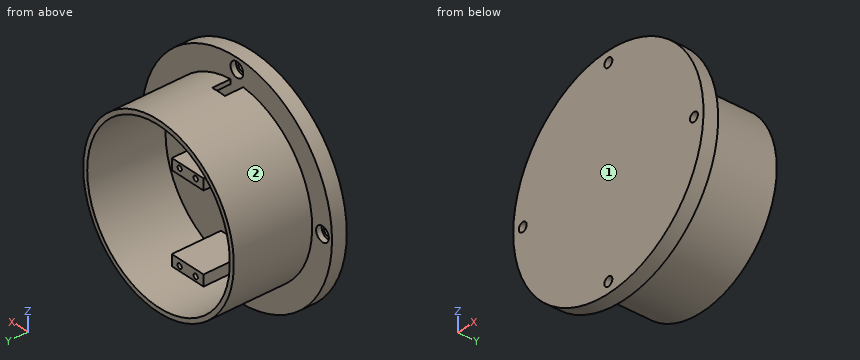
Autodesk Inventor part; units mm, degrees
ref_plane "YZ Plane" through (0, 0, 0) normal (1, 0, 0) x (0, 1, 0)
ref_plane "XZ Plane" through (0, 0, 0) normal (0, 1, 0) x (-1, 0, 0)
ref_plane "XY Plane" through (0, 0, 0) normal (0, 0, 1) x (1, 0, 0)
sketch "Sketch1" plane through (0, 0, 0) normal (0, 1, 0) x (-1, 0, 0)
  circle A0 centre (0, 0) radius 60
  dimension "d0" = 120
extrude "Extrusion1" add sketch "Sketch1" along normal blind 8
sketch "Sketch2" plane through (0, 8, 0) normal (0, 1, 0) x (1, 0, 0)
  circle A0 centre (-54, 0) radius 4
  circle A1 centre (-54, 0) radius 2.5
  circle A2 centre (0, -54) radius 4
  circle A3 centre (0, -54) radius 2.5
  circle A4 centre (54, 0) radius 4
  circle A5 centre (54, 0) radius 2.5
  circle A6 centre (0, 54) radius 4
  circle A7 centre (0, 54) radius 2.5
  point P0 (0, 0)
  dimension "d3" = 8
  dimension "d4" = 5
  dimension "d5" = 8
  dimension "d6" = 5
  dimension "d7" = 8
  dimension "d8" = 5
  dimension "d9" = 8
  dimension "d10" = 5
extrude "Extrusion2" cut sketch "Sketch2" against normal blind 8 contours A1 | A3 | A5 | A7
sketch "Sketch3" plane through (0, 8, 0) normal (0, 1, 0) x (1, 0, 0)
  circle A0 centre (-54, 0) radius 2.5
  circle A1 centre (-54, 0) radius 4
  circle A2 centre (-54, 0) radius 2.5
  circle A3 centre (0, 54) radius 2.5
  circle A4 centre (0, 54) radius 4
  circle A5 centre (0, 54) radius 2.5
  circle A6 centre (54, 0) radius 2.5
  circle A7 centre (54, 0) radius 4
  circle A8 centre (54, 0) radius 2.5
  circle A9 centre (0, -54) radius 4
  circle A10 centre (0, -54) radius 2.5
  point P0 (0, 0)
  dimension "d13" = 8
  dimension "d14" = 8
  dimension "d15" = 5
  dimension "d16" = 8
  dimension "d17" = 5
  dimension "d18" = 8
extrude "Extrusion3" cut sketch "Sketch3" against normal blind 3
sketch "Sketch4" plane through (0, 8, 0) normal (0, 1, 0) x (1, 0, 0)
  circle A0 centre (0, 0) radius 47.5
  circle A1 centre (0, 0) radius 45
  line L0 (0, 0) -> (-10, 0)
  line L1 (-10, 0) -> (-10, -9)
  line L2 (-10, -9) -> (0, -9)
  line L3 (0, -9) -> (0, 0)
  line L4 (0, -9) -> (10, -9)
  line L5 (10, -9) -> (10, 0)
  line L6 (10, 0) -> (0, 0)
  line L7 (0, 0) -> (0, -9)
  line L8 (-10, -9) -> (10, -9)
  line L9 (10, -9) -> (10, -16)
  line L10 (10, -16) -> (-10, -16)
  line L11 (-10, -16) -> (-10, -9)
  dimension "d21" = 95
  dimension "d22" = 90
  dimension "d23" = 10
  dimension "d24" = 9
  dimension "d25" = 10
  dimension "d26" = 7
extrude "Extrusion4" add sketch "Sketch4" along normal blind 10 contours A0
sketch "Sketch5" plane through (0, 8, 0) normal (0, 1, 0) x (1, 0, 0)
  line L0 (0, 0) -> (-10, 0)
  line L1 (-10, 0) -> (-10, -9)
  line L2 (-10, -9) -> (0, -9)
  line L3 (0, -9) -> (0, 0)
  line L4 (-10, -9) -> (10, -9)
  line L5 (10, -9) -> (10, -16)
  line L6 (10, -16) -> (-10, -16)
  line L7 (-10, -16) -> (-10, -9)
  line L8 (-10, -9) -> (10, -9)
  line L9 (10, -9) -> (10, 31)
  line L10 (10, 31) -> (-10, 31)
  line L11 (-10, 31) -> (-10, -9)
  line L12 (-10, 31) -> (-2, 31)
  line L13 (-2, 31) -> (-2, 38.36)
  line L14 (-2, 38.36) -> (-10, 38.36)
  line L15 (-10, 38.36) -> (-10, 31)
  line L16 (-10, 31) -> (10, 31)
  line L17 (10, 31) -> (10, 39)
  line L18 (10, 39) -> (-10, 39)
  line L19 (-10, 39) -> (-10, 31)
  line L20 (-10, -9) -> (10, -9)
  line L21 (10, -9) -> (10, -17)
  line L22 (10, -17) -> (-10, -17)
  line L23 (-10, -17) -> (-10, -9)
  dimension "d29" = 10
  dimension "d30" = 9
  dimension "d31" = 20
  dimension "d32" = 7
  dimension "d33" = 40
  dimension "d34" = 8
  dimension "d35" = 8
  dimension "d36" = 8
extrude "Extrusion5" add sketch "Sketch5" along normal blind 28 contours L4 L5 L6 L7 L2 | L15 L14 L13 L10 | L6 L21 L22 L23 | L13 L14 L19 L18 L17 L10
sketch "Sketch6" plane through (0, 36, 0) normal (0, 1, 0) x (1, 0, 0)
  line L0 (10, -17) -> (-10, -17)
  line L1 (-10, -9) -> (10, -9)
  line L2 (0, -17) -> (-4, -17)
  line L3 (-4, -17) -> (-4, -9)
  line L4 (-4, -9) -> (0, -9)
  line L5 (0, -9) -> (0, -17)
  line L6 (0, -17) -> (4, -17)
  line L7 (4, -17) -> (4, -9)
  line L8 (4, -9) -> (0, -9)
  line L9 (0, -9) -> (0, -17)
  point P0 (0, 0)
  dimension "d39" = 4
  dimension "d40" = 4
extrude "Extrusion6" cut sketch "Sketch6" against normal blind 28
sketch "Sketch7" plane through (0, 36, 0) normal (0, 1, 0) x (1, 0, 0)
  line L0 (-10, -17) -> (-4, -17)
  line L1 (4, -9) -> (10, -9)
  line L2 (-4, -17) -> (4, -17)
  line L3 (4, -17) -> (4, -9)
  line L4 (4, -9) -> (-4, -9)
  line L5 (-4, -9) -> (-4, -17)
  point P0 (0, 0)
extrude "Extrusion7" add sketch "Sketch7" against normal blind 22
sketch "Sketch8" plane through (0, 36, 0) normal (0, 1, 0) x (1, 0, 0)
  line L0 (-4, -17) -> (-10, -17)
  line L1 (10, -17) -> (10, -9)
  line L2 (-10, -17) -> (10, -17)
  line L3 (10, -17) -> (10, -15)
  line L4 (10, -15) -> (-10, -15)
  line L5 (-10, -15) -> (-10, -17)
  line L6 (-4, -9) -> (4, -9)
  line L7 (0, -9) -> (-5, -9)
  line L8 (-5, -9) -> (-5, -17)
  line L9 (-5, -17) -> (0, -17)
  line L10 (0, -17) -> (0, -9)
  line L11 (-10, -17) -> (10, -17)
  line L12 (0, -9) -> (5, -9)
  line L13 (5, -9) -> (5, -17)
  line L14 (5, -17) -> (0, -17)
  line L15 (0, -17) -> (0, -9)
  circle A0 centre (-5, -15) radius 2
  circle A1 centre (5, -15) radius 2
  line L16 (-10, 31) -> (-10, 39)
  line L17 (10, 39) -> (10, 31)
  line L18 (-10, 39) -> (10, 39)
  line L19 (10, 39) -> (10, 37)
  line L20 (10, 37) -> (-10, 37)
  line L21 (-10, 37) -> (-10, 39)
  line L22 (10, 31) -> (-10, 31)
  line L23 (-10, 39) -> (10, 39)
  line L24 (0, 31) -> (-5, 31)
  line L25 (-5, 31) -> (-5, 39)
  line L26 (-5, 39) -> (0, 39)
  line L27 (0, 39) -> (0, 31)
  line L28 (0, 31) -> (5, 31)
  line L29 (5, 31) -> (5, 39)
  line L30 (5, 39) -> (0, 39)
  line L31 (0, 39) -> (0, 31)
  circle A2 centre (-5, 37) radius 2
  circle A3 centre (5, 37) radius 2
  point P0 (0, 0)
  dimension "d45" = 2
  dimension "d46" = 5
  dimension "d47" = 5
  dimension "d48" = 4
  dimension "d49" = 4
  dimension "d50" = 2
  dimension "d51" = 4
  dimension "d52" = 4
extrude "Extrusion8" cut sketch "Sketch8" against normal blind 10 contours A0 L4 L8 | L8 L4 A0 | L8 A0 L4 | L4 A0 L8 | A1 L4 L13 | L13 L4 A1 | L13 A1 L4 | L4 A1 L13 | A2 L25 L20 | L20 L25 A2 | L25 L20 A2 | A2 L20 L25 | A3 L20 L29 | L29 L20 A3 | A3 L29 L20 | A3 L20 L29
sketch "Sketch9" plane through (0, 36, 0) normal (0, 1, 0) x (1, 0, 0)
  line L0 (-10, -17) -> (-5, -17)
  line L1 (10, -9) -> (-10, -9)
  line L2 (-10, -17) -> (10, -17)
  line L3 (10, -17) -> (10, -9)
  line L4 (10, -9) -> (-10, -9)
  line L5 (-10, -9) -> (-10, -17)
  line L6 (10, 31) -> (10, 39)
  line L7 (-10, 31) -> (10, 31)
  line L8 (10, 31) -> (10, 39)
  line L9 (10, 39) -> (-10, 39)
  line L10 (-10, 39) -> (-10, 31)
  point P0 (0, 0)
extrude "Extrusion9" cut sketch "Sketch9" against normal blind 28
sketch "Sketch10" plane through (0, 8, 0) normal (0, 1, 0) x (1, 0, 0)
  line L0 (0, 0) -> (-10, 0)
  line L1 (-10, 0) -> (-10, 36.5)
  line L2 (-10, 36.5) -> (0, 36.5)
  line L3 (0, 36.5) -> (0, 0)
  line L4 (-10, 0) -> (0, 0)
  line L5 (0, 0) -> (0, -16.9)
  line L6 (0, -16.9) -> (-10, -16.9)
  line L7 (-10, -16.9) -> (-10, 0)
  line L8 (0, -16.9) -> (10, -16.9)
  line L9 (10, -16.9) -> (10, 36.5)
  line L10 (10, 36.5) -> (0, 36.5)
  line L11 (0, 36.5) -> (0, -16.9)
  line L12 (-10, -16.9) -> (10, -16.9)
  line L13 (10, -16.9) -> (10, -10.9)
  line L14 (10, -10.9) -> (-10, -10.9)
  line L15 (-10, -10.9) -> (-10, -16.9)
  line L16 (-10, 36.5) -> (10, 36.5)
  line L17 (10, 36.5) -> (10, 30.5)
  line L18 (10, 30.5) -> (-10, 30.5)
  line L19 (-10, 30.5) -> (-10, 36.5)
  line L20 (-10, -16.9) -> (-4, -16.9)
  line L21 (-4, -16.9) -> (-4, -10.9)
  line L22 (-4, -10.9) -> (-10, -10.9)
  line L23 (-10, -10.9) -> (-10, -16.9)
  line L24 (10, -16.9) -> (4, -16.9)
  line L25 (4, -16.9) -> (4, -10.9)
  line L26 (4, -10.9) -> (10, -10.9)
  line L27 (10, -10.9) -> (10, -16.9)
  dimension "d57" = 10
  dimension "d58" = 36.5
  dimension "d59" = 16.9
  dimension "d60" = 10
  dimension "d61" = 6
  dimension "d62" = 6
  dimension "d63" = 6
  dimension "d64" = 6
extrude "Extrusion10" add sketch "Sketch10" along normal blind 10 contours L18 L1 L2 L3 | L3 L10 L9 L18 | L14 L21 L6 L7 | L14 L9 L8 L25
sketch "Sketch11" plane through (0, 18, 0) normal (0, 1, 0) x (1, 0, 0)
  line L0 (-10, 30.5) -> (10, 30.5)
  line L1 (10, 36.5) -> (-10, 36.5)
  line L2 (-10, 30.5) -> (10, 30.5)
  line L3 (10, 30.5) -> (10, 36.5)
  line L4 (10, 36.5) -> (-10, 36.5)
  line L5 (-10, 36.5) -> (-10, 30.5)
  line L6 (-10, -16.9) -> (-4, -16.9)
  line L7 (10, -10.9) -> (4, -10.9)
  line L8 (-10, -16.9) -> (10, -16.9)
  line L9 (10, -16.9) -> (10, -10.9)
  line L10 (10, -10.9) -> (-10, -10.9)
  line L11 (-10, -10.9) -> (-10, -16.9)
  point P0 (0, 0)
extrude "Extrusion11" add sketch "Sketch11" along normal blind 16.7
sketch "Sketch12" plane through (0, 34.7, 0) normal (0, 1, 0) x (1, 0, 0)
  line L0 (10, -16.9) -> (10, -10.9)
  line L1 (-10, -16.9) -> (10, -16.9)
  line L2 (10, -16.9) -> (10, -14.35)
  line L3 (10, -14.35) -> (-10, -14.35)
  line L4 (-10, -14.35) -> (-10, -16.9)
  line L5 (10, 30.5) -> (10, 36.5)
  line L6 (-10, 36.5) -> (10, 36.5)
  line L7 (10, 36.5) -> (10, 33.95)
  line L8 (10, 33.95) -> (-10, 33.95)
  line L9 (-10, 33.95) -> (-10, 36.5)
  line L10 (0, -16.9) -> (5.05, -16.9)
  line L11 (5.05, -16.9) -> (5.05, -14.35)
  line L12 (5.05, -14.35) -> (0, -14.35)
  line L13 (0, -14.35) -> (0, -16.9)
  line L14 (0, -16.9) -> (-5.05, -16.9)
  line L15 (-5.05, -16.9) -> (-5.05, -14.35)
  line L16 (-5.05, -14.35) -> (0, -14.35)
  line L17 (0, -14.35) -> (0, -16.9)
  line L18 (10, 36.5) -> (-10, 36.5)
  line L19 (0, 36.5) -> (-5.05, 36.5)
  line L20 (-5.05, 36.5) -> (-5.05, 33.95)
  line L21 (-5.05, 33.95) -> (0, 33.95)
  line L22 (0, 33.95) -> (0, 36.5)
  line L23 (0, 36.5) -> (5.05, 36.5)
  line L24 (5.05, 36.5) -> (5.05, 33.95)
  line L25 (5.05, 33.95) -> (0, 33.95)
  line L26 (0, 33.95) -> (0, 36.5)
  circle A0 centre (-5.05, -14.35) radius 1.35
  circle A1 centre (5.05, -14.35) radius 1.35
  circle A2 centre (-5.05, 33.95) radius 1.35
  circle A3 centre (5.05, 33.95) radius 1.35
  point P0 (0, 0)
  dimension "d69" = 2.55
  dimension "d70" = 2.55
  dimension "d71" = 5.05
  dimension "d72" = 5.05
  dimension "d73" = 5.05
  dimension "d74" = 5.05
  dimension "d75" = 2.7
  dimension "d76" = 2.7
  dimension "d77" = 2.7
  dimension "d78" = 2.7
extrude "Extrusion12" cut sketch "Sketch12" against normal blind 10 contours A1 L11 L3 | L3 A1 | A1 L3 L11 | A0 L3 L15 | L15 L3 A0 | L3 A0 | A3 L8 | L8 L24 A3 | L8 A3 L24 | A2 L8 | L8 L20 A2 | L20 L8 A2
thread "Thread1"
thread "Thread2"
thread "Thread3"
thread "Thread4"
sketch "Sketch13" plane through (0, 18, 0) normal (0, 1, 0) x (1, 0, 0)
  circle A0 centre (0, 0) radius 45
  circle A1 centre (0, 0) radius 47.5
extrude "Extrusion13" cut sketch "Sketch13" against normal blind 47.3
sketch "Sketch14" plane through (0, 8, 0) normal (0, 1, 0) x (1, 0, 0)
  circle A0 centre (0, 0) radius 45
  circle A1 centre (0, 0) radius 47.5
extrude "Extrusion14" add sketch "Sketch14" along normal blind 42.5
sketch "Sketch16" plane through (0, 50.5, 0) normal (0, 1, 0) x (1, 0, 0)
  circle A0 centre (0, 0) radius 45
  circle A1 centre (0, 0) radius 47.5
extrude "Extrusion15" cut sketch "Sketch16" against normal blind 42.5
sketch "Sketch17" plane through (0, 0, 0) normal (0, -1, 0) x (1, 0, 0)
  circle A0 centre (0, 0) radius 47.5
  circle A1 centre (0, 0) radius 45
extrude "Extrusion16" add sketch "Sketch17" against normal blind 8
sketch "Sketch18" plane through (0, 8, 0) normal (0, 1, 0) x (1, 0, 0)
  circle A0 centre (0, 0) radius 47.5
  circle A1 centre (0, 0) radius 45
  dimension "d97" = 95
  dimension "d98" = 90
extrude "Extrusion17" add sketch "Sketch18" along normal blind 42.5
sketch "Sketch19" plane through (4, 8, 16.9) normal (0, 0, 1) x (1, 0, 0)
  line L0 (-8, 0) -> (-8, 10)
  line L1 (-8, 0) -> (0, 0)
  line L2 (0, 0) -> (0, 10)
  line L3 (0, 10) -> (-8, 10)
  line L4 (-8, 10) -> (-8, 0)
  point P0 (-4, -8)
extrude "Extrusion18" add sketch "Sketch19" along normal blind 51.275
sketch "Sketch20" plane through (4, 8, 68.175) normal (0, 0, 1) x (1, 0, 0)
  line L0 (0, 0) -> (0, 10)
  line L1 (-8, 10) -> (0, 10)
  line L2 (0, 10) -> (0, 0)
  line L3 (0, 0) -> (-8, 0)
  line L4 (-8, 0) -> (-8, 10)
  point P0 (-4, -8)
extrude "Extrusion19" cut sketch "Sketch20" against normal blind 82.075
properties part number "NBase Part"
Design review of the part built by this model. Coordinates are the model's own, in mm. Face numbers are marked on the shaded views. A direction names the side the tool comes from. Round coordinates to 2 decimals unless told otherwise and drop trailing zeros. Write each loop counter-clockwise with the first axis right and the second up, starting at its lowest first coordinate (ties: lowest second). Pieces come first, ordered by that corner, then holes. Notation, with made-up numbers: (35, 51.5) - (70, 51.5) arc R21 cw to (70, 57.5) - close; hole circle Ø4 at (84, 51). An arc over 180 degrees is marked (long way). Use a Markdown table: item, result. Add a question column.
1. Wall thickness on probe 1 along Z at (x, y) = (0, 7); probe 2 along X at (y, z) = (29.25, 14.35); probe 3 along Y at (x, z) = (35.5, 25.5): over which ranges is each line inside the solid? List them lowest first.
2. For the marked faces 1 and 2, list the 3-axis set-ups (+Z, -Z, +X, -X, +Y, -Y) from which the entire face can be reached by the end or side of a thin tool; tool diameter is ignored.
3. We need section D-D (x = 0). Count the separate pieces of the cut face and the enclosed holes in it, then the cut area to 3 significant figures.
4. We need section A-A (y = 21). State the section outline as (x, z) points, then the cut area to 3 significant figures.
5. We need section B-B (y = 30). State the section outline as (x, z) points.
6. We need section C-C (z = 0). State the section outline as (x, y) points, then the cut area to 3 significant figures.
7. Clearance check with flat-ended pins moving along their axes: pin 1 (3 mm diameter, centred on x = -5.05, z = 14.35, fed in from +Y); pin 2 (4 mm diameter, centred on x = -55.5, z = 0, fed in from +Y); pin 3 (12 mm diameter, centred on y = 26.5, z = -2, fed in from +X); pin 4 (4 mm diameter, centred on x = 0, z = 54, fed in from +Y). State where each tip first meets the part, or that it passes through.
Output:
| question | item | result |
|---|---|---|
| 1 | probe 1 | z = -60 to -58, -50 to 50, 58 to 60 |
| 1 | probe 2 | x = -45.28 to -42.65, -10 to -6.4, -3.7 to 3.7, 6.4 to 10, 42.65 to 45.28 |
| 1 | probe 3 | y = 0 to 8 |
| 2 | face 1 | +Z, -Z, +X, -X, -Y |
| 2 | face 2 | +Y |
| 3 | separate pieces | 5 |
| 3 | enclosed holes | 0 |
| 3 | area | 1,310 mm2 |
| 4 | outline | circle Ø95 at (0, 0); (-10, -36.5) - (10, -36.5) - (10, -30.5) - (-10, -30.5) - close; (-10, 10.9) - (10, 10.9) - (10, 16.9) - (-10, 16.9) - close; hole circle Ø90 at (0, 0) |
| 4 | area | 966 mm2 |
| 5 | outline | circle Ø95 at (0, 0); (-10, -36.5) - (10, -36.5) - (10, -30.5) - (-10, -30.5) - close; (-10, 10.9) - (10, 10.9) - (10, 16.9) - (-10, 16.9) - close; hole circle Ø90 at (0, 0); hole circle Ø2.7 at (-5.05, -33.95); hole circle Ø2.7 at (-5.05, 14.35); hole circle Ø2.7 at (5.05, -33.95); hole circle Ø2.7 at (5.05, 14.35) |
| 6 | outline | (-60, 0) - (-56.5, 0) - (-56.5, 5) - (-58, 5) - (-58, 8) - (-60, 8) - close; (-51.5, 0) - (51.5, 0) - (51.5, 5) - (50, 5) - (50, 8) - (47.5, 8) - (47.5, 50.5) - (45, 50.5) - (45, 8) - (-45, 8) - (-45, 50.5) - (-47.5, 50.5) - (-47.5, 8) - (-50, 8) - (-50, 5) - (-51.5, 5) - close; (56.5, 0) - (60, 0) - (60, 8) - (58, 8) - (58, 5) - (56.5, 5) - close |
| 6 | area | 1,070 mm2 |
| 7 | pin 1 | stops at y = 34.7 |
| 7 | pin 2 | stops at y = 5 |
| 7 | pin 3 | stops at x = 47.5 |
| 7 | pin 4 | passes through |
